Autodesk Inventor part; units mm, degrees
ref_plane "YZ Plane" through (0, 0, 0) normal (1, 0, 0) x (0, 1, 0)
ref_plane "XZ Plane" through (0, 0, 0) normal (0, 1, 0) x (-1, 0, 0)
ref_plane "XY Plane" through (0, 0, 0) normal (0, 0, 1) x (1, 0, 0)
sketch "Sketch1" plane through (0, 0, 0) normal (0, 0, 1) x (1, 0, 0)
  line L0 (-13.3, 0) -> (13.3, 0)
  line L1 (0, -13.3) -> (0, 13.3)
  circle A0 centre (0, 0) radius 9.5
  circle A1 centre (0, 0) radius 1.3
  circle A2 centre (0, 0) radius 3.17
  dimension "d0" = 19
  dimension "d1" = 2.6
  dimension "d2" = 6.34
extrude "Extrusion4" add sketch "Sketch1" along normal mid plane 2.5 contours A1 L1 A2 L0 | L0 A2 L1 A1 | A2 L1 A0 L0 | L0 A0 L1 A2 | A1 L0 A2 L1 | L1 A2 L0 A1 | A2 L0 A0 L1 | L1 A0 L0 A2
sketch "Sketch3" plane through (0, 0, -1.25) normal (0, 0, -1) x (-1, 0, 0)
  circle A0 centre (0, 0) radius 3.175
  circle A1 centre (0, 0) radius 1.3021
  dimension "d21" = 6.35
extrude "Extrusion5" add sketch "Sketch3" along normal blind 7.36
sketch "Sketch4" plane through (0, 0, 1.25) normal (0, 0, 1) x (1, 0, 0)
  circle A0 centre (0, 0) radius 9.5
  line L0 (-5.6994, 7.6005) -> (5.6994, 7.6005)
  arc A1 (5.6994, 7.6005) -> (-5.6994, 7.6005) centre (0, 0) ccw
  dimension "d27" = 11.3988
sketch "Sketch5" plane through (0, 0, 1.25) normal (0, 0, 1) x (1, 0, 0)
  point P0 (0, 0)
  point P1 (0, 0)
hole "Hole1" at (0, 0, 1.25) direction (0, 0, -1) diameter 3.5 end through all
sketch "Sketch6" plane through (0, 0, 1.25) normal (0, 0, 1) x (1, 0, 0)
  circle A0 centre (0, 0) radius 6.35 construction
  circle A1 centre (0, -6.35) radius 1.585
  line L0 (0, -13.3) -> (0, 13.3) construction
  line L1 (-13.3, 0) -> (13.3, 0) construction
  circle A2 centre (5.4993, 3.175) radius 1.585
  circle A3 centre (-5.4993, 3.175) radius 1.585
  dimension "d40" = 12.7
  dimension "d41" = 3.17
  dimension "d44" = 360
extrude "Extrusion7" cut sketch "Sketch6" against normal through all
sketch "Sketch7" plane through (0, 0, 1.25) normal (0, 0, 1) x (1, 0, 0)
  circle A0 centre (0, 0) radius 9.5
properties part number "nakretka_na_igle"
CAD build for the part. Positions are in the model's coordinates, mm. A direction names the side the tool comes from. Coordinates: 2 decimals unless noted, no trailing zeros. Order: outer loops, then holes, each group sorted by start corner. A loop starts at its lowest first (then second) coordinate and runs counter-clockwise, first axis right, second up.
(1) Which spindle directions (+Z, -Z, +X, -X, +Y, -Y) get a long thin tool onto all of the face, cutting with end or side? Do faces 1 (the face through (4.38, -8.43, 0.02)), 2 (the face through (0, -4, -1.25)). Say none if no direction does.
Solution:
face 1: +Z, -Z
face 2: -Z
(2) Mould opens along X. For faces 3 (the face through (-4.77, 1.77, 0.02)), 4 (the face through (-1.4, -1.4, -8.61)), 5 (the face through (6.963, 2.568, 0.018)), 6 (the face through (0.69, 3.1, -4.88)) say: released by +X, released by -X, zero draft, split by the parting line, or undercut.
Solution:
face 3: undercut
face 4: zero draft
face 5: undercut
face 6: split by the parting line
(3) Drill centre lines: L1, parallel to Y at x = 0, z = 0.2 (3 decimals); L2, parallel to Y at x = 0, z = -6.5 (3 decimals); L3, parallel to Z at x = -1, y = 8. Where is each one in solid material? Low to high.
Solution:
L1: y = -9.5 to -7.935, -4.765 to -1.75, 1.75 to 9.5
L2: y = -3.175 to -1.75, 1.75 to 3.175
L3: z = -1.25 to 1.25
(4) Saw through at B-B, the plane x = 0. Write the cut outline in (y, z) (3 decimals).
Solution:
outline: (-9.5, -1.25) - (-7.935, -1.25) - (-7.935, 1.25) - (-9.5, 1.25) - close; (-4.765, -1.25) - (-3.175, -1.25) - (-3.175, -8.61) - (-1.75, -8.61) - (-1.75, 1.25) - (-4.765, 1.25) - close; (1.75, -8.61) - (3.175, -8.61) - (3.175, -1.25) - (9.5, -1.25) - (9.5, 1.25) - (1.75, 1.25) - close
(5) Pin check, flat tips, straight feed: pin 1 Ø1.5 at (x, y) = (6.5, -1) entering from -Z; pin 2 Ø1 at (y, z) = (0, -7) entering from +X (3 decimals); pin 3 Ø1.5 at (y, z) = (2.5, -7) entering from -X. Stop position of each tip, or through.
Solution:
pin 1: stops at z = -1.25
pin 2: stops at x = 3.175
pin 3: stops at x = -2.65
(6) Saw through at A-A, the plane y = 0. Write the cut outline in (x, z) (3 decimals).
Solution:
outline: (-9.5, -1.25) - (-3.175, -1.25) - (-3.175, -8.61) - (-1.75, -8.61) - (-1.75, 1.25) - (-9.5, 1.25) - close; (1.75, -8.61) - (3.175, -8.61) - (3.175, -1.25) - (9.5, -1.25) - (9.5, 1.25) - (1.75, 1.25) - close
(7) Saw through at C-C, the plane z = -0.75. Write the cut outline in (x, y) (3 decimals).
Solution:
outline: circle Ø19 at (0, 0); hole circle Ø3.17 at (-5.499, 3.175); hole circle Ø3.5 at (0, 0); hole circle Ø3.17 at (0, -6.35); hole circle Ø3.17 at (5.499, 3.175)
(8) Saw through at D-D, the plane y = 4.25. Write the cut outline in (x, z), and give its area (3 significant figures).
Solution:
outline: (-8.5, -1.25) - (-6.66, -1.25) - (-6.66, 1.25) - (-8.5, 1.25) - close; (-4.33, -1.25) - (4.33, -1.25) - (4.33, 1.25) - (-4.33, 1.25) - close; (6.66, -1.25) - (8.5, -1.25) - (8.5, 1.25) - (6.66, 1.25) - close
area: 30.8 mm2
